Build history of the part. All positions in model axes, mm. Face numbers are marked on the shaded views. A direction names the side the tool comes from. Coordinates: 2 decimals unless noted, no trailing zeros. Loops run counter-clockwise (first coordinate to the right, second up) from the corner with the lowest first, then second, coordinate; pieces in that order, holes last.
(1) Slice it at A-A (x = 58). Give the cut face in (y, z), and give its area (3 significant figures).
(2) Slice it at C-C (y = -21). Give the cut face in (x, z), and give its area (3 significant figures).
(3) Flat gauge pins, fed straight in: P1, Ø5, axis at x = 118, y = -34, coming from the -Z side; P2, Ø2, axis at x = 72, z = -31.5, coming from the +Y side; P3, Ø15, axis at x = -140.5, z = 3.5, coming from the -Y side. Where does each tip first touch, or does it go through?
(4) Slice it at B-B (x = 0). Give the cut face in (y, z), and give its area (3 significant figures).
(5) Wall check: L1, parallel to Y at x = -7.5, z = -67.5; L2, parallel to Z at x = -86, y = 40; L3, parallel to Y at x = -84, z = 8. Give the ranges that are in metal, low to high.
(6) Slice it at D-D (z = 27). Give the cut face in (x, y).
(7) Tool access for the marked faces 1, 2 and 3: list every direction of +Z, -Z, +X, -X, +Y, -Y with a clear straight run to the whole face (end or side of a thin tool).
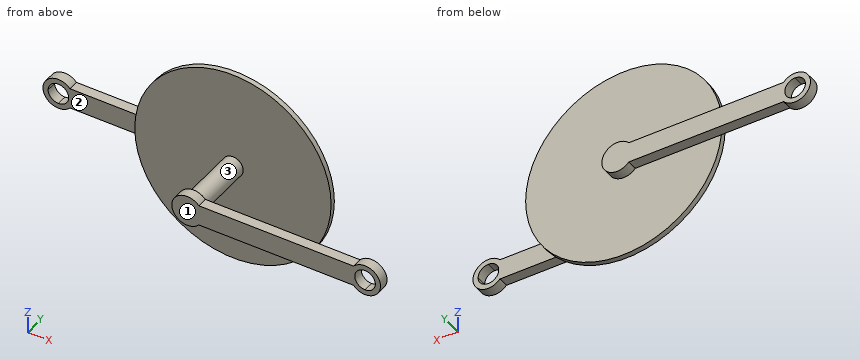
from build123d import *

# Parameters (mm, degrees)
F0_R     = 10
F1_DEPTH = 30
F3_DEPTH = 10
F4_R     = 95.25
F5_DEPTH = 5
F7_DEPTH = 10


with BuildPart() as f1:
    # F0 (on Front) → F1 (new body, symmetric)
    with BuildSketch(Plane.XZ):
        Circle(F0_R)
    extrude(amount=F1_DEPTH, both=True)

    # F2 (on face) → F3 (join)
    with BuildSketch(Plane.XZ.offset(30)):
        with BuildLine():
            ThreePointArc((11.180508, 9.999812), (-15, 0.000126), (11.18034, -10))
            Line((11.18034, -10), (161.31966, -10))
            ThreePointArc((161.31966, -10), (187.5, 0.000126), (161.319492, 9.999812))
            Line((161.319492, 9.999812), (11.180508, 9.999812))
        make_face()
        with BuildLine():
            ThreePointArc((172.561293, 9.999812), (179.592705, 7.049364), (182.5, 0))
            ThreePointArc((182.5, 0), (179.571068, -7.071068), (172.5, -10))
            ThreePointArc((172.5, -10), (162.500047, -0.030647), (172.438707, 9.999812))
            ThreePointArc((172.438707, 9.999812), (172.5, 10), (172.561293, 9.999812))
        make_face(mode=Mode.SUBTRACT)
    extrude(amount=F3_DEPTH)

    # F4 (on face) → F5 (join)
    with BuildSketch(Plane(origin=(0, 30, 0), x_dir=(-1, 0, 0), z_dir=(0, 1, 0))):
        Circle(F4_R)
    extrude(amount=F5_DEPTH)

    # F6 (on face) → F7 (join)
    with BuildSketch(Plane(origin=(0, 35, 0), x_dir=(-1, 0, 0), z_dir=(0, 1, 0))):
        with BuildLine():
            Line((161.319515, 9.999837), (11.180485, 9.999837))
            ThreePointArc((11.180485, 9.999837), (-15, 0.000109), (11.18034, -10))
            Line((11.18034, -10), (161.31966, -10))
            ThreePointArc((161.31966, -10), (187.5, 0.000109), (161.319515, 9.999837))
        make_face()
        with BuildLine():
            ThreePointArc((172.557026, 9.999837), (179.591201, 7.050877), (182.5, 0))
            ThreePointArc((182.5, 0), (179.571068, -7.071068), (172.5, -10))
            ThreePointArc((172.5, -10), (162.500041, -0.028513), (172.442974, 9.999837))
            ThreePointArc((172.442974, 9.999837), (172.5, 10), (172.557026, 9.999837))
        make_face(mode=Mode.SUBTRACT)
    extrude(amount=F7_DEPTH)


solid = f1.part
Response values:
1. outline: (-40, -10) - (-30, -10) - (-30, 10) - (-40, 10) - close; (30, -75.56) - (35, -75.56) - (35, 75.56) - (30, 75.56) - close
1. area: 956 mm2
2. outline: circle Ø20 at (0, 0)
2. area: 314 mm2
3. P1: stops at z = -10
3. P2: stops at y = 35
3. P3: stops at y = 35
4. outline: (-40, -15) - (-30, -15) - (-30, -10) - (30, -10) - (30, -95.25) - (35, -95.25) - (35, -15) - (45, -15) - (45, 15) - (35, 15) - (35, 95.25) - (30, 95.25) - (30, 10) - (-30, 10) - (-30, 15) - (-40, 15) - close
4. area: 2,750 mm2
5. L1: y = 30 to 35
5. L2: z = -10 to 10
5. L3: y = 30 to 45
6. outline: (-91.34, 30) - (91.34, 30) - (91.34, 35) - (-91.34, 35) - close
7. face 1: +Z, -Z, +X, -X, -Y
7. face 2: +Z, -Z, -X, -Y
7. face 3: none
